Source: CAD feature listing. Evaluate the final solid. Frame: model axes, mm. A direction names the side the tool comes from. Round coordinates to 2 decimals unless told otherwise and drop trailing zeros. Write each loop counter-clockwise with the first axis right and the second up, starting at its lowest first coordinate (ties: lowest second). Pieces come first, ordered by that corner, then holes.
Autodesk Inventor part; units mm, degrees
ref_plane "YZ Plane" through (0, 0, 0) normal (1, 0, 0) x (0, 1, 0)
ref_plane "XZ Plane" through (0, 0, 0) normal (0, 1, 0) x (-1, 0, 0)
ref_plane "XY Plane" through (0, 0, 0) normal (0, 0, 1) x (1, 0, 0)
sketch "Sketch1" plane through (0, 0, 0) normal (0, 1, 0) x (-1, 0, 0)
  circle A0 centre (0, 0) radius 3
  dimension "d0" = 6
extrude "Extrusion1" add sketch "Sketch1" along normal blind 5.5
sketch "Sketch2" plane through (0, 5.5, 0) normal (0, 1, 0) x (1, 0, 0)
  circle A0 centre (0, 0) radius 25
  dimension "d3" = 50
extrude "Extrusion2" add sketch "Sketch2" along normal blind 2
sketch "Sketch3" plane through (0, 7.5, 0) normal (0, 1, 0) x (1, 0, 0)
  circle A0 centre (0, 0) radius 13
  circle A1 centre (0, 0) radius 10
  dimension "d6" = 20
  dimension "d24" = 26
extrude "Extrusion3" add sketch "Sketch3" along normal blind 94
sketch "Sketch4" plane through (0, 0, 0) normal (0, -1, 0) x (1, 0, 0)
  circle A0 centre (0, 0) radius 1
  dimension "d9" = 2
extrude "Extrusion4" cut sketch "Sketch4" against normal through all
thread "Thread2"
sketch "Sketch5" plane through (0, 7.5, 0) normal (0, 1, 0) x (1, 0, 0)
  circle A0 centre (0, 0) radius 1
  circle A1 centre (0, 0) radius 20
  circle A2 centre (-20, 0) radius 1.5
  circle A3 centre (-10, -17.3205) radius 1.5
  circle A4 centre (10, -17.3205) radius 1.5
  circle A5 centre (20, 0) radius 1.5
  circle A6 centre (10, 17.3205) radius 1.5
  circle A7 centre (-10, 17.3205) radius 1.5
  dimension "d16" = 40
  dimension "d17" = 3
  dimension "d20" = 360
extrude "Extrusion5" cut sketch "Sketch5" against normal through all contours A1 A5 | A1 A5 | A6 A1 | A1 A6 | A4 A1 | A1 A4 | A7 A1 | A1 A7 | A3 A1 | A1 A3 | A2 A1 | A1 A2
properties part number "CylinderAttachment"
1) Pull-direction query (Z, two-part tool) for faces 1 (the face through (0, 4, -1)), 2 (the face through (-10.325, 6.514, 18.785)), 3 (the face through (-10.316, 53.842, -7.91)), 4 (the face through (0, 5.5, 5)); classes: released by +Z, released by -Z, zero draft, split by the parting line, or undercut.
Taken from the geometry:
face 1: undercut
face 2: undercut
face 3: split by the parting line
face 4: zero draft
2) Section query A-A on z = 0. Return the cut outline in (x, y), then the cut area to 3 significant figures.
Taken from the geometry:
outline: (-25, 5.5) - (-21.5, 5.5) - (-21.5, 7.5) - (-25, 7.5) - close; (-18.5, 5.5) - (-3, 5.5) - (-3, 0) - (-1, 0) - (-1, 7.5) - (-10, 7.5) - (-10, 101.5) - (-13, 101.5) - (-13, 7.5) - (-18.5, 7.5) - close; (1, 0) - (3, 0) - (3, 5.5) - (18.5, 5.5) - (18.5, 7.5) - (13, 7.5) - (13, 101.5) - (10, 101.5) - (10, 7.5) - (1, 7.5) - close; (21.5, 5.5) - (25, 5.5) - (25, 7.5) - (21.5, 7.5) - close
area: 670 mm2
3) Material intervals for line 1 (Z direction, x = 0, y = 69); line 2 (Z direction, x = -10, y = 7), sorted ascending.
Taken from the geometry:
line 1: z = -13 to -10, 10 to 13
line 2: z = -22.91 to -18.82, -15.82 to 15.82, 18.82 to 22.91
4) Section query D-D on x = 0. Return the cut outline in (y, z), then the cut area to 3 significant figures.
Taken from the geometry:
outline: (0, -3) - (5.5, -3) - (5.5, -25) - (7.5, -25) - (7.5, -13) - (101.5, -13) - (101.5, -10) - (7.5, -10) - (7.5, -1) - (0, -1) - close; (0, 1) - (7.5, 1) - (7.5, 10) - (101.5, 10) - (101.5, 13) - (7.5, 13) - (7.5, 25) - (5.5, 25) - (5.5, 3) - (0, 3) - close
area: 682 mm2
5) Reachability of faces 5 (the face through (11, 7.5, 11)), 6 (the face through (3, 3, 0)), 7 (the face through (23.846, 6.486, 7.509)) from +Z, -Z, +X, -X, +Y, -Y: full face, straight path, thin tool, end or side. Return the list, or none.
Taken from the geometry:
face 5: +Y
face 6: -Y
face 7: +Y, -Y
6) Contact query for flat-ended pins moving along their axis: P1, Ø2, axis at x = 9, y = 56, coming from the -Z side; P2, Ø12, axis at y = 59, z = -7.5, coming from the +X side; P3, Ø3, axis at x = -9, y = 22.5, coming from the -Z side; P4, Ø1.8, axis at x = 10, z = 17.32, coming from the +Y side. Output: stop coordinate, or through.
Taken from the geometry:
P1: stops at z = -10.25
P2: stops at x = 12.91
P3: stops at z = -10.62
P4: passes through
7) Section query C-C on y = 30. Return the cut outline in (x, z), then the cut area to 3 significant figures.
Taken from the geometry:
outline: circle Ø26 at (0, 0); hole circle Ø20 at (0, 0)
area: 217 mm2
8) Section query B-B on x = 20. Return the cut outline in (y, z), then the cut area to 3 significant figures.
Taken from the geometry:
outline: (5.5, -15) - (7.5, -15) - (7.5, -1.5) - (5.5, -1.5) - close; (5.5, 1.5) - (7.5, 1.5) - (7.5, 15) - (5.5, 15) - close
area: 54.0 mm2
